Build history of the part. All positions in model axes, mm. A direction names the side the tool comes from. Round coordinates to 2 decimals unless told otherwise and drop trailing zeros. Loops run counter-clockwise (first coordinate to the right, second up) from the corner with the lowest first, then second, coordinate; pieces in that order, holes last.
from build123d import *

# Parameters (mm, degrees)
CHAMFER1_SIZE      = 0.508
CHAMFER2_SIZE      = 1.524
CUT_EXTRUDE1_DEPTH = 33.0548
FILLET1_R          = 0.762


with BuildPart() as part:
    # Sketch1 → Revolve1 (revolve)
    with BuildSketch(Plane.XY):
        with BuildLine():
            Line((0, 35.0012), (0, -19.9898))
            Line((0, -19.9898), (-7.9375, -19.9898))
            Line((-7.9375, -19.9898), (-7.9375, -3.81))
            Line((-7.9375, -3.81), (-6.223, -3.81))
            Line((-6.223, -3.81), (-6.223, -1.27))
            ThreePointArc((-6.223, -1.27), (-6.594974388, -0.371974388), (-7.493, 0))
            Line((-7.493, 0), (-13.0048, 0))
            Line((-13.0048, 0), (-13.0048, 12.065))
            Line((-13.0048, 12.065), (-8.9408, 12.065))
            Line((-8.9408, 12.065), (-8.9408, 22.225))
            ThreePointArc((-8.9408, 22.225), (-6.9215, 25.0317), (-8.9408, 27.8384))
            Line((-8.9408, 27.8384), (-8.9408, 30.1752))
            Line((-8.9408, 30.1752), (-4.1148, 35.0012))
            Line((-4.1148, 35.0012), (0, 35.0012))
        make_face()
    revolve(axis=Axis((0, -19.9898, 0), (0, -1, 0)))

    # Chamfer1
    chamfer1_edges = [part.edges().sort_by_distance(p)[0] for p in [
        (13.0048, 12.065, 0),
        (13.0048, 0, 0),
    ]]
    chamfer(chamfer1_edges, length=CHAMFER1_SIZE)

    # Chamfer2
    chamfer2_edges = [part.edges().sort_by_distance(p)[0] for p in [
        (7.9375, -19.9898, 0),
    ]]
    chamfer(chamfer2_edges, length=CHAMFER2_SIZE)

    # Sketch2 → Cut-Extrude1 (cut, through all)
    with BuildSketch(Plane(origin=(0, 12.065, 0), x_dir=(1, 0, 0), z_dir=(0, 1, 0))):
        with BuildLine():
            Line((-10.922, 7.059372425), (-10.922, -7.059372425))
            ThreePointArc((-10.922, -7.059372425), (-13.0048, 0), (-10.922, 7.059372425))
        make_face()
        with BuildLine():
            Line((10.922, 7.059372425), (10.922, -7.059372425))
            ThreePointArc((10.922, -7.059372425), (13.0048, 0), (10.922, 7.059372425))
        make_face()
    extrude(amount=-CUT_EXTRUDE1_DEPTH, mode=Mode.SUBTRACT)

    # Fillet1
    fillet1_edges = [part.edges().sort_by_distance(p)[0] for p in [
        (8.9408, 12.065, 0),
    ]]
    fillet(fillet1_edges, radius=FILLET1_R)


solid = part.part
(1) Slice it at B-B on z = 0. List the corners of the cut face in (x, y) (1 decimal), plus the area to 3 significant figures.
Responses:
outline: (-10.9, 0) - (-7.5, 0) arc R1.3 cw to (-6.2, -1.3) - (-6.2, -3.8) - (-7.9, -3.8) - (-7.9, -18.5) - (-6.4, -20) - (6.4, -20) - (7.9, -18.5) - (7.9, -3.8) - (6.2, -3.8) - (6.2, -1.3) arc R1.3 cw to (7.5, 0) - (10.9, 0) - (10.9, 12.1) - (9.7, 12.1) arc R0.8 cw to (8.9, 12.8) - (8.9, 22.2) arc R3 cw to (8.9, 27.8) - (8.9, 30.2) - (4.1, 35) - (-4.1, 35) - (-8.9, 30.2) - (-8.9, 27.8) arc R3 cw to (-8.9, 22.2) - (-8.9, 12.8) arc R0.8 cw to (-9.7, 12.1) - (-10.9, 12.1) - close
area: 937 mm2
(2) Which spindle directions (+Z, -Z, +X, -X, +Y, -Y) get a long thin tool onto all of the face, cutting with end or side? Do faces 4 (the face through (-0.19, 11.93, -12.63)), 5 (the face through (5, -3.81, 4)), 6 (the face through (7.095, 29.023, 5.44)). Say none if no direction does.
Responses:
face 4: -Z, +Y
face 5: none
face 6: +Y
(3) Pin check, flat tips, straight feed: P1, Ø2, axis at y = -6, z = 0, coming from the +X side; P2, Ø12, axis at x = -1, y = 29.5, coming from the +Z side; P3, Ø1, axis at x = 4.5, y = -13.5, coming from the -Z side. Stop position of each tip, or through.
Responses:
P1: stops at x = 7.94
P2: stops at z = 8.94
P3: stops at z = -6.86
(4) Probe line 1 (Y direction, x = -1.75, z = 7); line 2 (Y direction, x = 0.25, z = -10.25) (3 decimals); line 3 (Z direction, x = -0.5, y = 4.5). List the from-to ranges inside material, lowest first.
Responses:
line 1: y = -19.19 to -3.81, -0.03 to 23.75, 26.32 to 31.9
line 2: y = 0 to 12.065
line 3: z = -13 to 13
(5) Slice it at C-C on y = 15.5. List the corners of the cut face in (x, z), plus the area to 3 significant figures.
Responses:
outline: circle Ø17.88 at (0, 0)
area: 251 mm2
(6) Pull direction Y, two halves, no side cores. Call faces 1 (the face through (7, 12.065, 7)), 2 (the face through (1.72, -11.04, 7.75)), 3 (the face through (1.349, -2.522, 6.075)): +Y half, -Y half, draft (parallel to the pull), parting line (faces both ways), or undercut.
Responses:
face 1: +Y half
face 2: draft
face 3: undercut
(7) Slice it at D-D on y = 31. List the corners of the cut face in (x, z).
Responses:
outline: circle Ø16.23 at (0, 0)
